Verification items for the finished model (mm, model axes). A direction names the side the tool comes from. Give positions to 0.01 mm unless a question says otherwise; leave off trailing zeros. Loops run counter-clockwise (first coordinate to the right, second up) from the corner with the lowest first, then second, coordinate; pieces in that order, holes last. Notation, with made-up numbers: (-35, 10.5) -> (-14, 10.5) arc R12 cw to (-14, 21.5) -> close; hole circle Ø10 at (34.25, 23). An arc over 180 degrees is marked (long way). Answer in a Markdown table with one row per item. Add a question column.
Q1. Section check A-A on z = 28.5. Enter the section's corners in (x, y).
Q2. Gauge pin test, flat ends, axial feed: P1, Ø6, axis at x = 8, z = 22, coming from the -Y side; P2, Ø6, axis at y = 10.5, z = 17.5, coming from the +X side; P3, Ø6, axis at y = 15, z = 10, coming from the -X side; P4, Ø12, axis at x = -17, z = 22.5, coming from the -Y side. Record the tip position at first contact, or that the pin passes through.
Q3. Material ranges on probe 1 along Y at (x, z) = (-13, 15); probe 2 along X at (y, z) = (9, 19), recorded low to high.
Q4. Section check B-B on x = -16. Enter the section's corners in (y, z), and give its area (3 significant figures).
Q5. Set-up check for faces 1 (the face through (32, 20.655, 16)), 2 (the face through (0, 10, 16)), 3 (the face through (43.279, 38, 16)): record each of +Z, -Z, +X, -X, +Y, -Y from which the full face is reachable in a straight line by a thin tool's end or side.
Q6. Section check C-C on y = 6.5. Enter the section's corners in (x, z), and give its area (3 significant figures).
```python
from build123d import *

# Parameters (mm, degrees)
F1_DEPTH = 25.4
F2_SCALE = 1.25


with BuildPart() as f1:
    # F0 (on Top) → F1 (new body)
    with BuildSketch(Plane.XY):
        Polygon((0, 16.5241323411), (0, 0), (16.2604935467, 0), (16.2604935467, 16.5241323411), (34.6229039133, 16.5241323411), (34.6229039133, 45.2440679073), (-19.1962253302, 45.2440679073), (-19.1962253302, 16.5241323411), align=None)
    extrude(amount=F1_DEPTH)


with BuildPart() as f1_1:
    # F2: moved
    add(f1.part.scale(F2_SCALE))


solid = f1_1.part
```
Taken from the geometry:
| question | item | result |
|---|---|---|
| 1 | outline | (-24, 20.66) -> (0, 20.66) -> (0, 0) -> (20.33, 0) -> (20.33, 20.66) -> (43.28, 20.66) -> (43.28, 56.56) -> (-24, 56.56) -> close |
| 2 | P1 | stops at y = 0 |
| 2 | P2 | stops at x = 20.33 |
| 2 | P3 | stops at x = 0 |
| 2 | P4 | stops at y = 20.66 |
| 3 | probe 1 | y = 20.66 to 56.56 |
| 3 | probe 2 | x = 0 to 20.33 |
| 4 | outline | (20.66, 0) -> (56.56, 0) -> (56.56, 31.75) -> (20.66, 31.75) -> close |
| 4 | area | 1,140 mm² |
| 5 | face 1 | +Z, -Z, +X, -Y |
| 5 | face 2 | +Z, -Z, -X, -Y |
| 5 | face 3 | +Z, -Z, +X, +Y, -Y |
| 6 | outline | (0, 0) -> (20.33, 0) -> (20.33, 31.75) -> (0, 31.75) -> close |
| 6 | area | 645 mm² |
